For this review, take the finished solid that the model builds, in its own axes (mm). Face numbers are marked on the shaded views. A direction names the side the tool comes from. Round coordinates to 2 decimals unless told otherwise and drop trailing zeros. Write each loop counter-clockwise with the first axis right and the second up, starting at its lowest first coordinate (ties: lowest second). Pieces come first, ordered by that corner, then holes. Notation, with made-up numbers: (47.25, 69.5) - (64.25, 69.5) arc R13 ccw to (64.25, 86.5) - close; hole circle Ø9 at (-33, -3.75). An arc over 180 degrees is marked (long way). One line per item, written item: value. Start each with the question number.
Q1. Add section A-A on z = 0. Write out the cut boundary in (x, y).
Q2. For probe 1 along Y at (x, z) = (93.5, 0); probe 2 along X at (y, z) = (0.5, -5); probe 3 along Y at (x, z) = (64, 1), list the stretches that pass through material, from the lowest coordinate up.
Q3. Tool access review of the marked faces 1 and 2: name each direction out of +Z, -Z, +X, -X, +Y, -Y from which nothing blocks a thin tool from reaching the whole face with its end or side.
Q4. Add section C-C on x = 60. Write out the cut boundary in (y, z), and give its area (3 significant figures).
Q5. Add section B-B on y = 0. Write out the cut boundary in (x, z), and give its area (3 significant figures).
Q6. Clearance check with flat-ended pins moving along their axes: pin 1 Ø2 at (x, z) = (2, 6) entering from -Y; pin 2 Ø12 at (x, z) = (41.5, -10) entering from +Y; pin 3 Ø1.5 at (x, z) = (63.5, 10) entering from -Y. State where each tip first meets the part, or that it passes through.
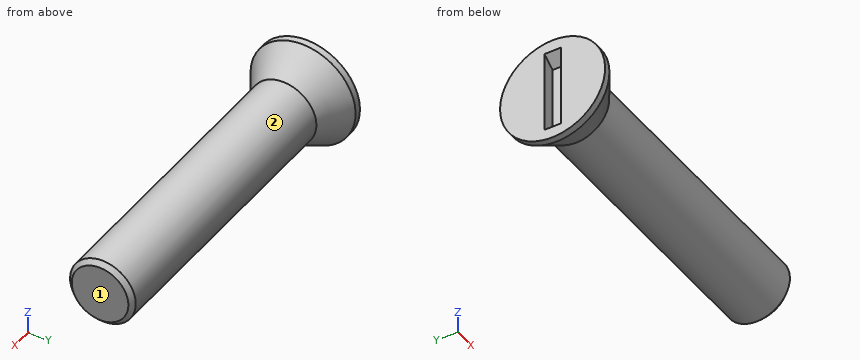
```python
from build123d import *

# Parameters (mm, degrees)
SLOT_DEPTH      = 2.5
SLOT_DEPTH_BACK = 2.5


with BuildPart() as part:
    # BodySke → BaseBody (revolve)
    with BuildSketch(Plane.XY, mode=Mode.PRIVATE) as basebody_sk:
        Polygon((0, 0), (0, 16), (2.081886537, 16), (11.5, 10), (98.626, 10), (100, 8.626), (100, 0), align=None)
    revolve(basebody_sk.sketch.rotate(Axis((0, 0, 0), (1, 0, 0)), 90), axis=Axis((0, 0, 0), (1, 0, 0)))

    # SlotSke → Slot (cut, two sides: drawn at the far end of the back side and taken through both)
    with BuildSketch(Plane(origin=(0, 0, 0), x_dir=(1, 0, 0), z_dir=(0, 1, 0)).offset(-SLOT_DEPTH_BACK)):
        Polygon((0, 12.5), (4, 9.951718957), (4, -9.951718957), (0, -12.5), align=None)
    extrude(amount=SLOT_DEPTH + SLOT_DEPTH_BACK, mode=Mode.SUBTRACT)


solid = part.part
```
Result set:
1. outline: (0, -16) - (2.08, -16) - (11.5, -10) - (98.63, -10) - (100, -8.63) - (100, 8.63) - (98.63, 10) - (11.5, 10) - (2.08, 16) - (0, 16) - (0, 2.5) - (4, 2.5) - (4, -2.5) - (0, -2.5) - close
2. probe 1: y = -10 to 10
2. probe 2: x = 4 to 100
2. probe 3: y = -9.95 to 9.95
3. face 1: +Z, -Z, +X, +Y, -Y
3. face 2: +X
4. outline: circle Ø20 at (0, 0)
4. area: 314 mm^2
5. outline: (0, -16) - (2.08, -16) - (11.5, -10) - (98.63, -10) - (100, -8.63) - (100, 8.63) - (98.63, 10) - (11.5, 10) - (2.08, 16) - (0, 16) - (0, 12.5) - (4, 9.95) - (4, -9.95) - (0, -12.5) - close
5. area: 1,990 mm^2
6. pin 1: stops at y = -15.2
6. pin 2: stops at y = 9.17
6. pin 3: stops at y = -3.8
